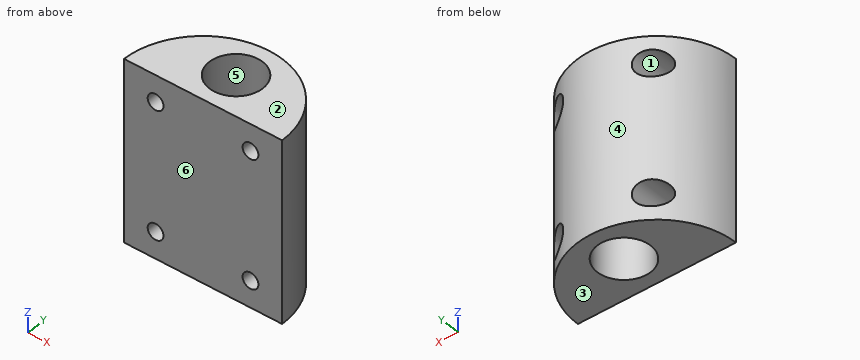
```python
from build123d import *

# Parameters (mm, degrees)
ESQUISSE1_R               = 5
BOSS_EXTRU_1_DEPTH        = 34
ESQUISSE2_R               = 1.5
ENL_V_MAT_EXTRU_1_DEPTH   = 48.759815745
ENL_V_START               = -5
ESQUISSE4_R               = 2.5
ENL_V_MAT_EXTRU_2_DEPTH   = 43.75981591
SYM_TRIE2_START           = -5
SYM_TRIE2_COPY_1_SKETCH_R = 2.5
SYM_TRIE2_COPY_1_DEPTH    = 43.75981591


with BuildPart() as part:
    # Esquisse1 → Boss.-Extru.1 (new body)
    with BuildSketch(Plane.XY):
        with BuildLine():
            Line((0, 0), (30, 0))
            ThreePointArc((30, 0), (15, 15), (0, 0))
        make_face()
        with Locations((15, 7.5)):
            Circle(ESQUISSE1_R, mode=Mode.SUBTRACT)
    extrude(amount=BOSS_EXTRU_1_DEPTH)

    # Esquisse2 → Enlèv. mat.-Extru.1 (cut, through all)
    with BuildSketch(Plane.XZ):
        with Locations(Location((24, 29, 0), (0, 0, 270))):
            Circle(ESQUISSE2_R)
        with Locations(Location((24, 5, 0), (0, 0, 270))):
            Circle(ESQUISSE2_R)
        with Locations(Location((6, 5, 0), (0, 0, 270))):
            Circle(ESQUISSE2_R)
        with Locations(Location((6, 29, 0), (0, 0, 270))):
            Circle(ESQUISSE2_R)
    extrude(amount=-ENL_V_MAT_EXTRU_1_DEPTH, mode=Mode.SUBTRACT)

    # Esquisse4 → Enlèv. mat.-Extru.2 (cut, through all)
    with BuildSketch(Plane.XZ.offset(ENL_V_START)):
        with Locations(Location((24, 29, 0), (0, 0, 270))):
            Circle(ESQUISSE4_R)
    enl_v_mat_extru_2 = extrude(amount=-ENL_V_MAT_EXTRU_2_DEPTH, mode=Mode.SUBTRACT)

    # Symétrie1: Enlèv. mat.-Extru.2 across plane
    add(enl_v_mat_extru_2.mirror(Plane(origin=(15, 0, 0), x_dir=(0, 0, 1), z_dir=(1, 0, 0))), mode=Mode.SUBTRACT)

    # Symétrie2: Enlèv. mat.-Extru.2 across plane
    add(enl_v_mat_extru_2.mirror(Plane.XY.offset(17)), mode=Mode.SUBTRACT)

    # Symétrie2 copy 1 sketch → Symétrie2 copy 1 (cut, through all)
    with BuildSketch(Plane(origin=(30, 0, 34), x_dir=(-1, 0, 0), z_dir=(0, -1, 0)).offset(SYM_TRIE2_START)):
        with Locations(Location((24, 29, 0), (0, 0, 270))):
            Circle(SYM_TRIE2_COPY_1_SKETCH_R)
    extrude(amount=-SYM_TRIE2_COPY_1_DEPTH, mode=Mode.SUBTRACT)


solid = part.part
```
Here's how the part is built. I have some questions about the finished solid (model axes, mm). Face numbers are marked on the shaded views. A direction names the side the tool comes from. Round coordinates to 2 decimals unless told otherwise and drop trailing zeros. Order: outer loops, then holes, each group sorted by start corner. A loop starts at its lowest first (then second) coordinate and runs counter-clockwise, first axis right, second up. Notation, with made-up numbers: M 42.25,62 L 95.25,62 A12 cw 95.25,70 Z; hole C -31.75,27 d2. An arc over 180 degrees is marked long. Use CSV: the item, a comma, the result in double quotes.
1) I want a section at C-C (x = 6). List the corners of the cut face in (y, z) for me.
Taken from the geometry:
outline,"M 0,0 L 12,0 L 12,2.5 L 5,2.5 L 5,3.5 L 0,3.5 Z; M 0,6.5 L 5,6.5 L 5,7.5 L 12,7.5 L 12,26.5 L 5,26.5 L 5,27.5 L 0,27.5 Z; M 0,30.5 L 5,30.5 L 5,31.5 L 12,31.5 L 12,34 L 0,34 Z"
2) I want a section at D-D (x = 15). List the corners of the cut face in (y, z) for me.
Taken from the geometry:
outline,"M 0,0 L 2.5,0 L 2.5,34 L 0,34 Z; M 12.5,0 L 15,0 L 15,34 L 12.5,34 Z"
3) I'm going to push flat-ended pins straight in: P1, Ø1, axis at y = 12, z = 14, coming from the +X side; P2, Ø6, axis at y = 10, z = 30, coming from the -X side; P3, Ø4, axis at x = 23.5, z = 5.5, coming from the +Y side; P4, Ø4, axis at x = 13, z = 19, coming from the +Y side. Where does each tip first touch, or does it pass through?
Taken from the geometry:
P1,"x = 24.63"
P2,"x = 1.73"
P3,"y = 13.52"
P4,"y = 15"
4) If we mould it in two halves opening along Y, with no side actions, what happens to the marked faces 3, 4, 5 and 6? For each: pulls with the +Y half, pulls with the -Y half, needs draft (parallel to the pull), parting line crosses it, or undercut.
Taken from the geometry:
face 3,"needs draft"
face 4,"pulls with the +Y half"
face 5,"undercut"
face 6,"pulls with the -Y half"
5) I need wall thicknesses on line 1 along X through (y, z) = (1.2, 29); line 2 along X through (y, z) = (10.5, 27); line 3 along X through (y, z) = (8, 5). Which ranges of each line are inside material? Lowest first, please. Write a range as [from, to].
Taken from the geometry:
line 1,"[0.05, 4.5], [7.5, 22.5], [25.5, 29.95]"
line 2,"[4.29, 4.5], [7.5, 11], [19, 22.5], [25.5, 25.71]"
line 3,"[2.31, 3.5], [8.5, 10.03], [19.97, 21.5], [26.5, 27.69]"
6) On a 3-axis mill with a long thin cutter (end or side, diameter ignored), from which of +Z, -Z, +X, -X, +Y, -Y can I reach the whole of each face in a straight line? I mean the marked faces 1 and 2. Say none if no direction works.
Taken from the geometry:
face 1,"+Y"
face 2,"+Z, +X, -X, +Y, -Y"
7) I want a section at A-A (z = 5). List the corners of the cut face in (x, y) for me, then the cut area to 3 significant figures.
Taken from the geometry:
outline,"M 0,0 L 4.5,0 L 4.5,5 L 3.5,5 L 3.5,9.63 A15 ccw Z; M 7.5,0 L 22.5,0 L 22.5,5 L 21.5,5 L 21.5,13.52 A15 ccw 8.5,13.52 L 8.5,5 L 7.5,5 Z; M 25.5,0 L 30,0 A15 ccw 26.5,9.63 L 26.5,5 L 25.5,5 Z; hole C 15,7.5 d10"
area,"176 mm^2"
8) I want a section at B-B (y = 7.5). List the corners of the cut face in (x, z) for me.
Taken from the geometry:
outline,"M 2.01,0 L 10,0 L 10,34 L 2.01,34 Z; M 20,0 L 27.99,0 L 27.99,34 L 20,34 Z; hole C 6,5 d5; hole C 6,29 d5; hole C 24,5 d5; hole C 24,29 d5"
